Part model, mm, in its own coordinate system. A direction names the side the tool comes from. Coordinates: 2 decimals unless noted, no trailing zeros. Loops run counter-clockwise (first coordinate to the right, second up) from the corner with the lowest first, then second, coordinate; pieces in that order, holes last. Notation, with made-up numbers: M 18,9 L 53,9 A15 ccw 53,32 Z; hole C 80.5,-38 d11. An arc over 180 degrees is marked long. Answer as a JSON object with one key per item and string values. Group by question number.
1. Saw through at D-D on x = 43. Count the separate pieces of the cut face and the enclosed holes in it, then the cut area to 3 significant figures.
2. Drop flat-ended pins along their axis: pin 1 Ø19.5 at (y, z) = (108.56, -44.97) entering from -X; pin 2 Ø1.5 at (y, z) = (43.5, 90.5) entering from +X; pin 3 Ø10 at (x, y) = (55.5, 17.5) entering from +Z; pin 4 Ø4 at (x, z) = (19, 67.5) entering from +Y. Give the stop position or say it passes through.
3. 3-axis set-ups, long thin cutter, end or side, ignore diameter. For faces 5 (the face through (28.94, -28.73, 109.27)), 6 (the face through (60.88, -10.349, 78.823)), 7 (the face through (7, 62, -62)): which of +Z, -Z, +X, -X, +Y, -Y reach the whole face in a straight line?
4. Saw through at A-A on z = 0. Write the cut outline in (x, y).
5. Drill centre lines: L1, parallel to Y at x = 37.5, z = -95; L2, parallel to Y at x = 39.5, z = 37; L3, parallel to Z at x = 28, y = 0.5. Where is each one in solid material? Low to high.
6. Saw through at C-C on x = 59. Write the cut outline in (y, z), then the cut area to 3 significant figures.
7. Mould opens along Y. For faces 1 (the face through (28.94, 28.73, -109.27)), 2 (the face through (51.5, 62, -62)), 3 (the face through (3.549, -17.071, -76.877)), 4 (the face through (28.94, -109.27, -28.73)) say: released by +Y, released by -Y, zero draft, split by the parting line, or undercut.
Autodesk Inventor part; units mm, degrees
ref_plane "YZ Plane" through (0, 0, 0) normal (1, 0, 0) x (0, 1, 0)
ref_plane "XZ Plane" through (0, 0, 0) normal (0, 1, 0) x (-1, 0, 0)
ref_plane "XY Plane" through (0, 0, 0) normal (0, 0, 1) x (1, 0, 0)
sketch "Sketch1" plane through (0, 0, 0) normal (0, 0, 1) x (1, 0, 0)
  line L0 (0, 0) -> (70, 0) construction
  line L1 (0, 58) -> (0, 78.75)
  line L2 (0, 78.75) -> (7, 78.75)
  line L3 (7, 145) -> (51.5, 145)
  line L4 (0, 58) -> (0, 0) construction
  line L5 (7, 145) -> (7, 78.75)
  line L6 (51.5, 145) -> (51.5, 79.5)
  line L7 (0, 58) -> (70, 58)
  line L8 (70, 58) -> (70, 0) construction
  line L9 (51.5, 79.5) -> (70, 79.5)
  line L10 (70, 79.5) -> (70, 58)
  dimension "d0" = 157.5
  dimension "d1" = 290
  dimension "d2" = 159
  dimension "d3" = 7
  dimension "d8" = 70
  dimension "d9" = 116
  dimension "d10" = 44.5
revolve "Revolution1" add sketch "Sketch1" angle 360 about axis through (0, 0, 0) along (1, 0, 0)
sketch "Sketch2" plane through (7, 0, 0) normal (-1, 0, 0) x (0, 0, 1)
  circle A0 centre (0, 0) radius 78.75
  line L0 (0, 0) -> (0, 117.5) construction
  circle A1 centre (0, 0) radius 145
  circle A2 centre (0, 0) radius 117.5 construction
  line L1 (0, 0) -> (44.9653, 108.5558) construction
  circle A3 centre (44.9653, 108.5558) radius 16.25
  dimension "d12" = 32.5
  dimension "d13" = 235
  dimension "d14" = 22.5
extrude "Extrusion1" cut sketch "Sketch2" against normal blind 44.5 contours A3
pattern_circular "Circular Pattern1" count 8 over 360 about axis through (3.5, 0, 0) along (1, 0, 0) of "Extrusion1"
equation "\"d0\" = D1"
equation "\"d1\" = D"
equation "\"d2\" = N2"
equation "\"d3\" = F2"
equation "\"d8\" = H1"
equation "\"d9\" = B1"
equation "\"d10\" = C2"
equation "\"d12\" = L"
equation "\"d13\" = K1"
equation "\"d4\" = C2"
equation "\"C2\" = 44.5"
equation "\"D\" = 290"
equation "\"K1\" = 235"
equation "\"L\" = 32.5"
equation "\"N2\" = 159"
equation "\"D1\" = 157.5"
equation "\"H1\" = 70"
equation "\"F2\" = 7"
equation "\"B1\" = 116"
equation "\"Size_Designation\" = 1.2345"
properties part number "ISO 7005-1 Hubbed Slip-On Flange for Welding Type 12 - ISO PN 150 DN100" material "Steel"
Outcome:
{
 "1": {"separate pieces": "1", "enclosed holes": "9", "area": "48,800 mm²"},
 "2": {"pin 1": "passes through", "pin 2": "stops at x = 51.5", "pin 3": "stops at z = 144.27", "pin 4": "stops at y = 129.36"},
 "3": {"face 5": "+X, -X", "face 6": "+X", "face 7": "-X"},
 "4": {"outline": "M 0,-78.75 L 7,-78.75 L 7,-145 L 51.5,-145 L 51.5,-79.5 L 70,-79.5 L 70,-58 L 0,-58 Z; M 0,58 L 70,58 L 70,79.5 L 51.5,79.5 L 51.5,145 L 7,145 L 7,78.75 L 0,78.75 Z"},
 "5": {"L1": "y = -109.54 to -53.93, -36 to 36, 53.93 to 109.54", "L2": "y = -140.2 to -122.72, -94.39 to -44.67, 44.67 to 94.39, 122.72 to 140.2", "L3": "z = -145 to -58, 58 to 145"},
 "6": {"outline": "C 0,0 d159; hole C 0,0 d116", "area": "9,290 mm²"},
 "7": {"face 1": "undercut", "face 2": "zero draft", "face 3": "split by the parting line", "face 4": "undercut"}
}
